Could you check a few things on this model? Use its own coordinates, in mm. Coordinates: 2 decimals unless noted, no trailing zeros. Write each loop counter-clockwise with the first axis right and the second up, starting at its lowest first coordinate (ties: lowest second). Pieces come first, ordered by that corner, then holes. Notation, with made-up numbers: M 56.5,27 L 85.5,27 A17 ccw 85.5,48 Z; hole C 29.5,-0.75 d4. An arc over 180 degrees is marked long. Write item = value, one per line.
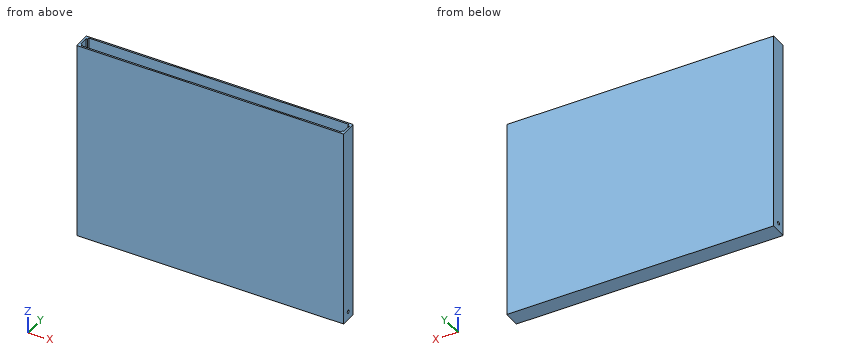
```python
from build123d import *

# Parameters (mm, degrees)
SKETCH1_W           = 508
SKETCH1_H           = 381
BOSS_EXTRUDE1_DEPTH = 31.75
SKETCH2_W           = 501.65
SKETCH2_H           = 25.4
CUT_EXTRUDE1_DEPTH  = 342.9
SKETCH3_W           = 3.175
SKETCH3_H           = 3.81
BOSS_EXTRUDE2_DEPTH = 35.56
SKETCH4_R           = 3.175
CUT_EXTRUDE2_DEPTH  = 25.4
CUT_EXTRUDE3_START  = -482.6
SKETCH4_2_R         = 3.175
CUT_EXTRUDE3_DEPTH  = 25.4


with BuildPart() as part:
    # Sketch1 → Boss-Extrude1 (new body)
    with BuildSketch(Plane(origin=(0, 0, 0), x_dir=(1, 0, 0), z_dir=(0, 1, 0))):
        Rectangle(SKETCH1_W, SKETCH1_H)
    extrude(amount=BOSS_EXTRUDE1_DEPTH)

    # Sketch2 → Cut-Extrude1 (cut)
    with BuildSketch(Plane.XY.offset(190.5)):
        with Locations((0, 15.875)):
            Rectangle(SKETCH2_W, SKETCH2_H)
    extrude(amount=-CUT_EXTRUDE1_DEPTH, mode=Mode.SUBTRACT)

    # Sketch3 → Boss-Extrude2 (add)
    with BuildSketch(Plane.XY.offset(190.5)):
        with Locations((-249.2375, 26.67)):
            Rectangle(SKETCH3_W, SKETCH3_H)
        with Locations((-249.2375, 5.08)):
            Rectangle(SKETCH3_W, SKETCH3_H)
        with Locations((249.2375, 5.08)):
            Rectangle(SKETCH3_W, SKETCH3_H)
        with Locations((249.2375, 26.67)):
            Rectangle(SKETCH3_W, SKETCH3_H)
    extrude(amount=-BOSS_EXTRUDE2_DEPTH)

    # Sketch4 → Cut-Extrude2 (cut)
    with BuildSketch(Plane.ZY.offset(254)):
        with Locations((-175.26, 15.24)):
            Circle(SKETCH4_R)
    extrude(amount=-CUT_EXTRUDE2_DEPTH, mode=Mode.SUBTRACT)

    # Sketch4<2> → Cut-Extrude3 (cut)
    with BuildSketch(Plane.ZY.offset(254).offset(CUT_EXTRUDE3_START)):
        with Locations((-175.26, 15.24)):
            Circle(SKETCH4_2_R)
    extrude(amount=-CUT_EXTRUDE3_DEPTH, mode=Mode.SUBTRACT)


solid = part.part
```
Item 1: I'm going to push flat-ended pins straight in: P1, Ø5, axis at y = 15.24, z = -175.26, coming from the +X side; P2, Ø3, axis at y = 15, z = -174, coming from the -X side. Where does each tip first touch, or does it pass through?
Numbers:
P1 = 228.6
P2 = -228.6
Item 2: If I drill on line 1 along Y through (x, z) = (241, -175); line 2 along X through (y, z) = (17, 69.5) (3 decimals); line 3 along Y through (x, z) = (3.5, 36.5) (3 decimals), over which ranges is the centre line in solid material (lowest first)?
Numbers:
line_1 = 0 to 12.08, 18.4 to 31.75
line_2 = -254 to -250.825, 250.825 to 254
line_3 = 0 to 3.175, 28.575 to 31.75
Item 3: Imagine slicing it at A-A (z = 35.5). Write out the boundary of the cut face in (x, y) (3 decimals).
Numbers:
outline = M -254,0 L 254,0 L 254,31.75 L -254,31.75 Z; hole M -250.825,3.175 L 250.825,3.175 L 250.825,28.575 L -250.825,28.575 Z
Item 4: Imagine slicing it at B-B (x = 78). Write out the boundary of the cut face in (y, z) (3 decimals), and give its area (3 significant figures).
Numbers:
outline = M 0,-190.5 L 31.75,-190.5 L 31.75,190.5 L 28.575,190.5 L 28.575,-152.4 L 3.175,-152.4 L 3.175,190.5 L 0,190.5 Z
area = 3,390 mm²
